Build history of the part. All positions in model axes, mm. A direction names the side the tool comes from. Round coordinates to 2 decimals unless told otherwise and drop trailing zeros. Loops run counter-clockwise (first coordinate to the right, second up) from the corner with the lowest first, then second, coordinate; pieces in that order, holes last.
from build123d import *

# Parameters (mm, degrees)
BOSS_EXTRUDE1_DEPTH = 55
SKETCH7_W           = 30
SKETCH7_H           = 45
CUT_EXTRUDE5_DEPTH  = 20
CUT_EXTRUDE4_REACH  = 74.457
SKETCH6_R           = 4.5
SKETCH8_R           = 8.75
BOSS_EXTRUDE2_DEPTH = 5
CUT_EXTRUDE6_REACH  = 71.642
SKETCH9_R           = 4.5


with BuildPart() as part:
    # Sketch1 → Boss-Extrude1 (new body)
    with BuildSketch(Plane(origin=(0, 0, 0), x_dir=(1, 0, 0), z_dir=(0, 1, 0))):
        Polygon((0, 0), (0, -40), (25, -40), (25, -30), (5, 0), align=None)
    extrude(amount=BOSS_EXTRUDE1_DEPTH)

    # Sketch7 → Cut-Extrude5 (cut)
    with BuildSketch(Plane(origin=(25, 0, 0), x_dir=(0, 0, -1), z_dir=(1, 0, 0))):
        with Locations((-15, 27.5)):
            Rectangle(SKETCH7_W, SKETCH7_H)
    extrude(amount=-CUT_EXTRUDE5_DEPTH, mode=Mode.SUBTRACT)

    # Sketch6 → Cut-Extrude4 (cut, up to next)
    with BuildSketch(Plane.XY.offset(40), mode=Mode.PRIVATE) as cut_extrude4_sk1:
        with Locations((15, 40)):
            Circle(SKETCH6_R)
    cut_extrude4_tool1 = extrude(cut_extrude4_sk1.sketch, amount=-CUT_EXTRUDE4_REACH, mode=Mode.PRIVATE) & part.part
    # Sketch6 → Cut-Extrude4 (cut, up to next)
    with BuildSketch(Plane.XY.offset(40), mode=Mode.PRIVATE) as cut_extrude4_sk2:
        with Locations((15, 15)):
            Circle(SKETCH6_R)
    cut_extrude4_tool2 = extrude(cut_extrude4_sk2.sketch, amount=-CUT_EXTRUDE4_REACH, mode=Mode.PRIVATE) & part.part
    add(cut_extrude4_tool1.solids().sort_by_distance((15, 40, 40))[0], mode=Mode.SUBTRACT)
    add(cut_extrude4_tool2.solids().sort_by_distance((15, 15, 40))[0], mode=Mode.SUBTRACT)

    # Sketch8 → Boss-Extrude2 (add)
    with BuildSketch(Plane(origin=(5, 0, 0), x_dir=(0, 0, -1), z_dir=(1, 0, 0))):
        with Locations((-10, 27.5)):
            Circle(SKETCH8_R)
    extrude(amount=BOSS_EXTRUDE2_DEPTH)

    # Sketch9 → Cut-Extrude6 (cut, up to next)
    with BuildSketch(Plane(origin=(10, 0, 0), x_dir=(0, 0, -1), z_dir=(1, 0, 0)), mode=Mode.PRIVATE) as cut_extrude6_sk1:
        with Locations((-10, 27.5)):
            Circle(SKETCH9_R)
    cut_extrude6_tool1 = extrude(cut_extrude6_sk1.sketch, amount=-CUT_EXTRUDE6_REACH, mode=Mode.PRIVATE) & part.part
    add(cut_extrude6_tool1.solids().sort_by_distance((10, 27.5, 10))[0], mode=Mode.SUBTRACT)


solid = part.part
(1) Slice it at B-B on y = 27.5. List the corners of the cut face in (x, z), plus the area to 4 significant figures.
Responses:
outline: (0, 0) - (5, 0) - (5, 1.25) - (10, 1.25) - (10, 5.5) - (0, 5.5) - close; (0, 14.5) - (10, 14.5) - (10, 18.75) - (5, 18.75) - (5, 30) - (25, 30) - (25, 40) - (0, 40) - close
area: 397.5 mm2
(2) Probe line 1 (Y direction, x = 15, z = 32.75); line 2 (Y direction, x = 10.25, z = 19.5); line 3 (Y direction, x = 6.5, z = 10). List the from-to ranges inside material, lowest first.
Responses:
line 1: y = 0 to 10.5, 19.5 to 35.5, 44.5 to 55
line 2: y = 0 to 5, 50 to 55
line 3: y = 0 to 5, 18.75 to 23, 32 to 36.25, 50 to 55
(3) Pull direction Z, two halves, no side cores. Call faces 1 (the face through (12, 27, 40)), 2 (the face through (11, 50, 22)), 3 (the face through (5, 33, 19)), 4 (the face through (15, 52, 15)): +Z half, -Z half, draft (parallel to the pull), parting line (faces both ways), or undercut.
Responses:
face 1: +Z half
face 2: draft
face 3: undercut
face 4: -Z half
(4) Slice it at A-A on x = 8.5. List the corners of the cut face in (y, z).
Responses:
outline: (0, 5.25) - (5, 5.25) - (5, 30) - (50, 30) - (50, 5.25) - (55, 5.25) - (55, 40) - (0, 40) - close; circle Ø17.5 at (27.5, 10); hole circle Ø9 at (27.5, 10)
(5) Slice it at D-D on x = 16. List the corners of the cut face in (y, z).
Responses:
outline: (0, 16.5) - (5, 16.5) - (5, 30) - (10.61, 30) - (10.61, 40) - (0, 40) - close; (19.39, 30) - (35.61, 30) - (35.61, 40) - (19.39, 40) - close; (44.39, 30) - (50, 30) - (50, 16.5) - (55, 16.5) - (55, 40) - (44.39, 40) - close
(6) Slice it at C-C on z = 7.5. List the corners of the cut face in (x, y), plus the area to 3 significant figures.
Responses:
outline: (0, 0) - (10, 0) - (10, 5) - (5, 5) - (5, 19.11) - (10, 19.11) - (10, 23.76) - (0, 23.76) - close; (0, 31.24) - (10, 31.24) - (10, 35.89) - (5, 35.89) - (5, 50) - (10, 50) - (10, 55) - (0, 55) - close
area: 334 mm2
(7) Which spindle directions (+Z, -Z, +X, -X, +Y, -Y) get a long thin tool onto all of the face, cutting with end or side? Do faces 5 (the face through (15, 2, 15)), 6 (the face through (14.41, 19.46, 35.07)), 7 (the face through (7.46, 18.96, 11.9)), 8 (the face through (10, 32, 12)). Say none if no direction does.
Responses:
face 5: -Z, +X, -Y
face 6: +Z, -Z
face 7: +X
face 8: -Z, +X
(8) Pin check, flat tips, straight feed: P1, Ø12, axis at y = 8, z = 16.5, coming from the +X side; P2, Ø24, axis at y = 31.5, z = 13, coming from the +X side; P3, Ø10, axis at x = 16, y = 22, coming from the -Z side. Stop position of each tip, or through.
Responses:
P1: stops at x = 19.46
P2: stops at x = 10
P3: stops at z = 30
